For this review, take the finished solid that the model builds, in its own axes (mm). A direction names the side the tool comes from. Round coordinates to 2 decimals unless told otherwise and drop trailing zeros. Use one line per item in the form item = value. Start each with the question number.
Autodesk Inventor part; units mm, degrees
ref_plane "YZ Plane" through (0, 0, 0) normal (1, 0, 0) x (0, 1, 0)
ref_plane "XZ Plane" through (0, 0, 0) normal (0, 1, 0) x (-1, 0, 0)
ref_plane "XY Plane" through (0, 0, 0) normal (0, 0, 1) x (1, 0, 0)
sketch "Sketch1" plane through (0, 0, 0) normal (0, 1, 0) x (-1, 0, 0)
  line L0 (-4.4, 0) -> (4.4, 0) construction
  line L1 (0, 0) -> (0, -12) construction
  line L2 (2.65, -12) -> (-2.65, -12) construction
  line L3 (2.65, -12) -> (4.4, 0)
  line L4 (-2.65, -12) -> (-4.4, 0)
  line L5 (0, -12) -> (0, -15.5) construction
  line L6 (0, -15.5) -> (-4, -15.5) construction
  line L7 (0, -15.5) -> (4, -15.5) construction
  line L8 (0, -15.5) -> (4, -15.5) construction
  line L9 (2.65, -12) -> (2.1396, -15.5)
  line L10 (-2.65, -12) -> (-2.1396, -15.5)
  line L11 (2.1396, -15.5) -> (-2.1396, -15.5)
  line L12 (-7.4, 0) -> (12.6, 0) construction
  line L13 (4.4, 0) -> (-4.4, 0)
  dimension "d0" = 8.8
  dimension "d1" = 12
  dimension "d2" = 5.3
  dimension "d3" = 3.5
  dimension "d4" = 4
  dimension "d5" = 4
  dimension "d7" = 3
sketch "Sketch2" plane through (0, 0, 0) normal (0, 1, 0) x (-1, 0, 0)
  line L0 (7.4, -46.26) -> (-7.4, -46.26)
  line L1 (-7.4, -46.26) -> (-7.4, 0)
  line L2 (-7.4, 0) -> (7.4, 0)
  line L3 (7.4, 0) -> (7.4, -46.26)
  line L4 (0, 0) -> (0, 4) construction
  line L5 (0, 0) -> (0, -46.26) construction
  dimension "d18" = 4
  dimension "d19" = 50.26
  dimension "d20" = 14.8
extrude "Extrusion1" add sketch "Sketch2" along normal mid plane 6
extrude "Extrusion2" cut sketch "Sketch1" along normal mid plane 2.4
sketch "Sketch3" plane through (0, 0, 0) normal (0, 1, 0) x (-1, 0, 0)
  line L0 (0, 0) -> (0, 4) construction
  line L1 (0, 0) -> (0, -46.26) construction
  dimension "d15" = 4
  dimension "d17" = 50.26
sketch "Sketch4" plane through (7.4, 3, -46.26) normal (0, 0, -1) x (-1, 0, 0)
  line L0 (-13.95, 5) -> (18.25, 5)
  line L1 (18.25, 5) -> (18.25, -11)
  line L2 (18.25, -11) -> (-13.95, -11)
  line L3 (-13.95, -11) -> (-13.95, 5)
  line L4 (-9.35, 3.1) -> (13.65, 3.1)
  line L5 (13.65, 3.1) -> (13.65, -9.1)
  line L6 (13.65, -9.1) -> (-9.35, -9.1)
  line L7 (-9.35, -9.1) -> (-9.35, 3.1)
  line L8 (2.15, 5) -> (2.15, -11) construction
  line L9 (18.25, -3) -> (-13.95, -3) construction
  line L10 (-9.35, 3.1) -> (-9.35, 5)
  line L11 (13.65, 3.1) -> (13.65, 5)
  line L12 (13.65, -9.1) -> (13.65, -11)
  line L13 (-9.35, -9.1) -> (-9.35, -11)
  circle A0 centre (16.15, -3) radius 1
  circle A1 centre (-11.85, -3) radius 1
  point P0 (7.4, -3)
  point P1 (2.15, -3)
  dimension "d21" = 32.2
  dimension "d22" = 16
  dimension "d23" = 23
  dimension "d24" = 12.2
  dimension "d25" = 2.5
  dimension "d26" = 2
  dimension "d27" = 2.5
  dimension "d28" = 2
  dimension "d43" = 5.25
extrude "Extrusion3" add sketch "Sketch4" along normal blind 15.72 and the other way blind 2 contours L0 L10 L7 L13 L2 L3 | L0 L1 L2 L12 L5 L11
extrude "Extrusion4" add sketch "Sketch4" along normal blind 4 and the other way blind 2 contours L0 L11 L4 L10 | L13 L6 L12 L2
extrude "Extrusion5" add sketch "Sketch4" against normal blind 2 contours A0 | A1
extrude "Extrusion6" add sketch "Sketch4" against normal blind 2 contours L4 L5 L6 L7
sketch "Sketch5" plane through (-10.85, -8, -61.98) normal (-1, 0, 0) x (0, 0, 1)
  line L0 (15.72, 1.9) -> (15.72, 14.1)
  line L1 (15.72, 8) -> (6.72, 8) construction
  line L2 (15.72, 6) -> (6.72, 6)
  line L3 (6.72, 6) -> (6.72, 10)
  line L4 (6.72, 10) -> (15.72, 10)
  line L5 (15.72, 10) -> (15.72, 6)
  line L6 (15.72, 6) -> (6.72, 10) construction
  line L7 (6.72, 6) -> (15.72, 10) construction
  point P0 (61.98, 8)
  point P1 (11.22, 8)
  dimension "d44" = 9
  dimension "d45" = 4
extrude "Extrusion7" cut sketch "Sketch5" against normal blind 6
sketch "Sketch6" plane through (-6.25, -8, -61.98) normal (1, 0, 0) x (0, 0, -1)
  line L0 (-15.72, 10) -> (-6.72, 10)
  line L1 (0, 0) -> (0, 16)
  line L2 (-6.72, 10) -> (0, 10)
  line L3 (0, 10) -> (0, 6)
  line L4 (0, 6) -> (-6.72, 6)
  line L5 (-6.72, 6) -> (-6.72, 10)
  point P0 (-61.98, 8)
  dimension "d48" = 4
extrude "Extrusion8" cut sketch "Sketch6" against normal blind 1
ref_plane "Work Plane1" through (7.4, 3, -32.26) normal (0, 0, 1) x (1, 0, 0)
sketch "Sketch7" plane through (7.4, 3, -32.26) normal (0, 0, 1) x (1, 0, 0)
  line L0 (-14.8, 0) -> (0, 0)
  line L1 (0, 0) -> (0, -6)
  line L2 (0, -6) -> (-14.8, -6)
  line L3 (-14.8, 0) -> (-14.8, -6)
  point P0 (-7.4, -3)
sketch "Sketch8" plane through (7.4, 3, -44.26) normal (0, 0, 1) x (1, 0, 0)
  line L0 (13.95, 5) -> (-18.25, 5)
  line L1 (-18.25, 5) -> (-18.25, -11)
  line L2 (-18.25, -11) -> (13.95, -11)
  line L3 (13.95, -11) -> (13.95, 5)
  point P0 (-7.4, -3)
loft "Loft1" add profiles "Sketch7" section 2 edges at (5.25, 8, -44.26) (-10.85, 0, -44.26) (5.25, -8, -44.26) (21.35, 0, -44.26)
properties part number "tilt_pillar"
Item 1: Take a section at A-A on y = 0. Give the number of separate pieces and of enclosed holes in the cut face, plus the area to 3 significant figures.
Item 2: Machinability: for faces 1 (the flat face through (-8, 2, -52)), 2 (the flat face through (-6.25, 5, -54)), 3 (the flat face through (0, -3, -16)), 4 (the flat face through (-7.4, 0, -16)), 5 (the flat face through (0, 1.2, -6)), which of the approach directions +Z, -Z, +X, -X, +Y, -Y give a long, thin tool a straight path to every point of the face, cutting with its end or side? Answer none if there is none.
Item 3: Wall thickness on line 1 (X direction, y = 3.25, z = -54); line 2 (Y direction, x = 19.25, z = -51); line 3 (Y direction, x = 14, z = -50): over which ranges is each line inside the solid? List them lowest first.
Item 4: For P1, Ø3, axis at x = 19.25, y = 0, coming from the -Z side; P2, Ø0.6, axis at x = 19, y = 0, coming from the -Z side; P3, Ø3, axis at x = 10.5, y = -6, coming from the +Z side; P4, Ø4.5, axis at x = 0.5, z = -9, coming from the -Y side, all flat-tipped, find the tip position at first contact; note any pin that passes through.
Item 5: Draft analysis for pull direction Z (two halves, no side actions). For faces 6 (the flat face through (5, -8, -49)), 7 (the flat face through (0.1, -1.4, 0)), 8 (the flat face through (-10, 0, -55.26)), state which applies: +Z half, -Z half, draft (parallel to the pull), parting line (faces both ways), or undercut.
Results:
q1.separate_pieces = 3
q1.enclosed_holes = 0
q1.area = 774 mm2
q2.face_1 = none
q2.face_2 = -Z
q2.face_3 = +Z, +X, -X, -Y
q2.face_4 = +Z, -X, +Y, -Y
q2.face_5 = +Z
q3.line_1 = -10.85 to -6.25, 16.75 to 21.35
q3.line_2 = -8 to -1, 1 to 8
q3.line_3 = -8 to -6.1, 6.1 to 8
q4.P1 = -61.98
q4.P2 = -46.26
q4.P3 = -35.86
q4.P4 = -3
q5.face_6 = draft
q5.face_7 = +Z half
q5.face_8 = undercut
